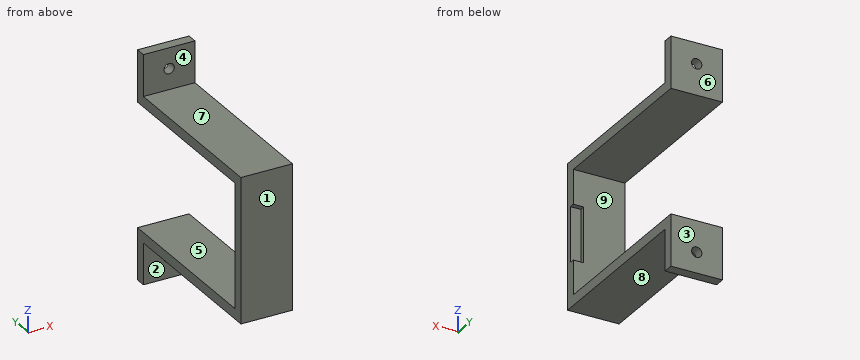
from build123d import *

# Parameters (mm, degrees)
EXTRUDE_1_DEPTH     = 15
CUT_EXTRUDE_1_REACH = 63.758
SKETCH_2_R          = 1.5
SKETCH_3_W          = 16
SKETCH_3_H          = 1.5
CUT_EXTRUDE_2_DEPTH = 3


with BuildPart() as part:
    # 草图1 → 凸台-拉伸1 (new body)
    with BuildSketch(Plane(origin=(0, 0, 0), x_dir=(0, 0, -1), z_dir=(1, 0, 0))):
        Polygon((0, 0), (18, 0), (18, 50), (33, 50), (33, 47), (21, 47), (21, -3), (0, -3), (-21, -3), (-21, 47), (-33, 47), (-33, 50), (-18, 50), (-18, 0), align=None)
    extrude(amount=EXTRUDE_1_DEPTH)

    # 草图2 → 切除-拉伸1 (cut, up to next)
    with BuildSketch(Plane.XZ.offset(-47), mode=Mode.PRIVATE) as cut_extrude_1_sk1:
        with Locations(Location((7.5, -27, 0), (0, 0, 270))):
            Circle(SKETCH_2_R)
    cut_extrude_1_tool1 = extrude(cut_extrude_1_sk1.sketch, amount=-CUT_EXTRUDE_1_REACH, mode=Mode.PRIVATE) & part.part
    # 草图2 → 切除-拉伸1 (cut, up to next)
    with BuildSketch(Plane.XZ.offset(-47), mode=Mode.PRIVATE) as cut_extrude_1_sk2:
        with Locations(Location((7.5, 27, 0), (0, 0, 270))):
            Circle(SKETCH_2_R)
    cut_extrude_1_tool2 = extrude(cut_extrude_1_sk2.sketch, amount=-CUT_EXTRUDE_1_REACH, mode=Mode.PRIVATE) & part.part
    add(cut_extrude_1_tool1.solids().sort_by_distance((7.5, 47, -27))[0], mode=Mode.SUBTRACT)
    add(cut_extrude_1_tool2.solids().sort_by_distance((7.5, 47, 27))[0], mode=Mode.SUBTRACT)

    # 草图3 → 切除-拉伸2 (cut)
    with BuildSketch(Plane(origin=(15, 0, 0), x_dir=(0, 0, -1), z_dir=(1, 0, 0))):
        with Locations((0, -0.75)):
            Rectangle(SKETCH_3_W, SKETCH_3_H)
    extrude(amount=-CUT_EXTRUDE_2_DEPTH, mode=Mode.SUBTRACT)


solid = part.part
CAD build for the part. Positions are in the model's coordinates, mm. Face numbers are marked on the shaded views. A direction names the side the tool comes from. Round coordinates to 2 decimals unless told otherwise and drop trailing zeros. Order: outer loops, then holes, each group sorted by start corner. A loop starts at its lowest first (then second) coordinate and runs counter-clockwise, first axis right, second up. Notation, with made-up numbers: (89, 44.5) -> (131, 44.5) arc R26 cw to (131, 72.5) -> close; hole circle Ø10 at (-18, 44). An arc over 180 degrees is marked (long way). Write item = value, one per line. Start each with the question number.
(1) Cut at D-D, the plane x = 2. List the corners of the cut face in (y, z), then the cut area to 3 significant figures.
(2) Pin check, flat tips, straight feed: P1, Ø6, axis at x = 10.5, z = 13, coming from the +Y side; P2, Ø1.2, axis at x = 13, y = -1, coming from the +Z side; P3, Ø3.5, axis at x = 14, z = 0, coming from the +Y side. Stop position of each tip, or through.
(3) Cut at B-B, the plane x = 7.5. List the corners of the cut face in (y, z).
(4) Cut at C-C, the plane z = -27. List the corners of the cut face in (x, y).
(5) Pull direction Z, two halves, no side cores. Call the marked faces 6, 7, 8 and 9: released by +Z, released by -Z, zero draft, split by the parting line, or undercut.
(6) Which spindle directions (+Z, -Z, +X, -X, +Y, -Y) get a long thin tool onto all of the face, cutting with end or side? Do the marked faces 1, 2, 3, 4 and 5. Say none if no direction does.
(7) Cut at A-A, the plane y = 41. List the corners of the cut face in (x, z), then the cut area to 3 significant figures.
(8) Probe line 1 (Z direction, x = 6, y = 18); line 2 (X direction, y = 48, z = -27); line 3 (Y direction, x = 8.25, z = 0). List the from-to ranges inside material, lowest first. Write a range as [from, to].
Model answer:
q1.outline = (-3, -21) -> (47, -21) -> (47, -33) -> (50, -33) -> (50, -18) -> (0, -18) -> (0, 18) -> (50, 18) -> (50, 33) -> (47, 33) -> (47, 21) -> (-3, 21) -> close
q1.area = 498 mm2
q2.P1 = 0
q2.P2 = 21
q2.P3 = -1.5
q3.outline = (-3, -21) -> (47, -21) -> (47, -25.5) -> (50, -25.5) -> (50, -18) -> (0, -18) -> (0, 18) -> (50, 18) -> (50, 25.5) -> (47, 25.5) -> (47, 21) -> (-3, 21) -> close; (47, -33) -> (50, -33) -> (50, -28.5) -> (47, -28.5) -> close; (47, 28.5) -> (50, 28.5) -> (50, 33) -> (47, 33) -> close
q4.outline = (0, 47) -> (6, 47) -> (6, 50) -> (0, 50) -> close; (9, 47) -> (15, 47) -> (15, 50) -> (9, 50) -> close
q5.face_6 = zero draft
q5.face_7 = released by +Z
q5.face_8 = released by -Z
q5.face_9 = undercut
q6.face_1 = +Z, -Z, +X, -X, -Y
q6.face_2 = -Z, +X, -X, -Y
q6.face_3 = +Z, -Z, +X, -X, +Y
q6.face_4 = +Z, +X, -X, -Y
q6.face_5 = +X, -X, +Y
q7.outline = (0, -21) -> (15, -21) -> (15, -18) -> (0, -18) -> close; (0, 18) -> (15, 18) -> (15, 21) -> (0, 21) -> close
q7.area = 90.0 mm2
q8.line_1 = [-21, -18], [18, 21]
q8.line_2 = [0, 6], [9, 15]
q8.line_3 = [-3, 0]
